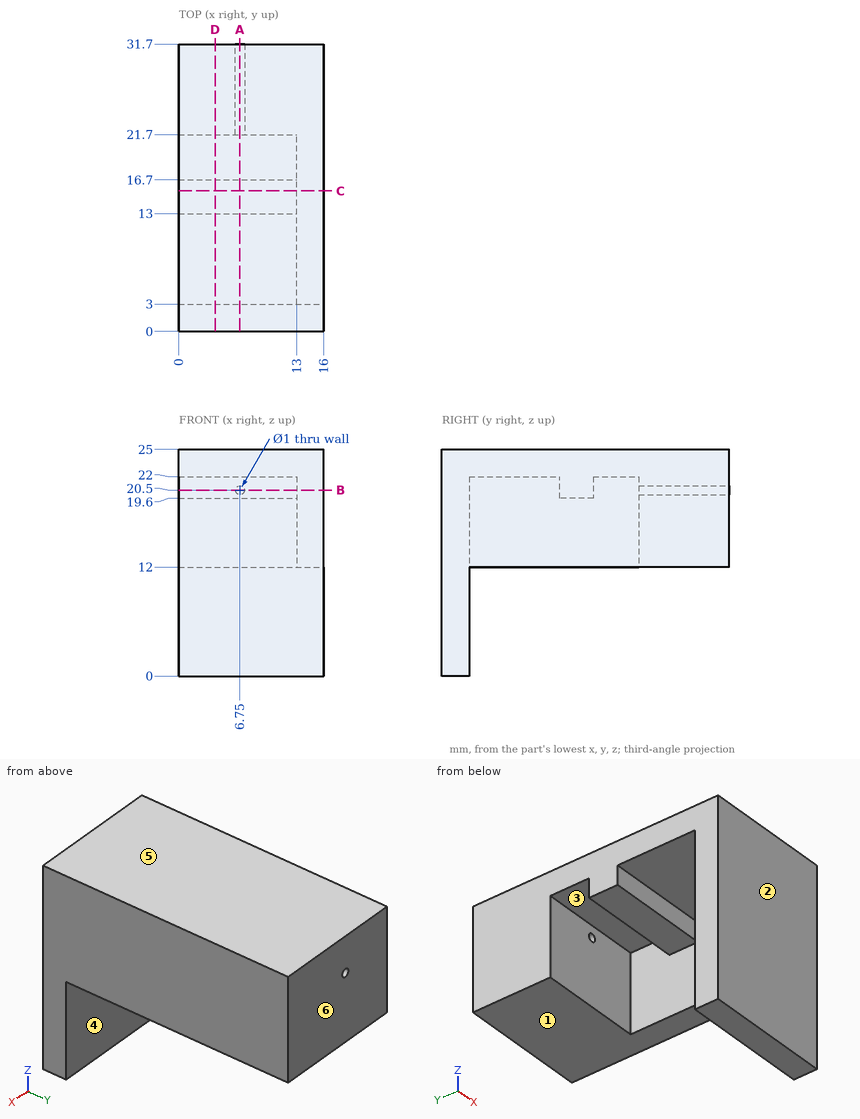
Can you work these out from the drawing? Everything is in mm from the part's minimum corner. A direction names the side the tool comes from. Give positions to 0.01 mm unless a question says otherwise; leave off trailing zeros. Order: outer loops, then holes, each group sorted by start corner. A loop starts at its lowest first (then second) coordinate and runs counter-clockwise, first axis right, second up. Notation, with made-up numbers: (-21.5, 17.5) -> (22.5, 17.5) arc R14 cw to (22.5, 40.5) -> close; hole circle Ø9 at (45, 70). An arc over 180 degrees is marked (long way). Return JSON: item names as keys, results as strings.
1. Imagine slicing it at C-C on y = 15.5. List the corners of the cut face in (x, z) for me.
Answer list:
{"outline": "(0, 19.6) -> (13, 19.6) -> (13, 12) -> (16, 12) -> (16, 25) -> (0, 25) -> close"}
2. For pin 1 Ø4 at (x, y) = (9, 15) entering from -Z; pin 2 Ø8 at (x, y) = (12.5, 18) entering from -Z; pin 3 Ø1 at (x, y) = (5.5, 11) entering from -Z, each with a flat end and sliding along its axis, tell me the tip position at first contact or that it passes through.
Answer list:
{"pin 1": "stops at z = 19.6", "pin 2": "stops at z = 12", "pin 3": "stops at z = 22"}
3. Thinking about a two-plate mould opening in Y: for the marked faces 4, 5 and 6, which applies, pulls with the +Y half, pulls with the -Y half, needs draft (parallel to the pull), parting line crosses it, or undercut?
Answer list:
{"face 4": "undercut", "face 5": "needs draft", "face 6": "pulls with the +Y half"}
4. I need wall thicknesses on line 1 (Y direction, x = 9.5, z = 20); line 2 (X direction, y = 25, z = 20.5); line 3 (Z direction, x = 6.75, y = 24). Which ranges of each line are inside material? Lowest first, please. Write a range as from..to.
Answer list:
{"line 1": "y = 0..3, 13..16.7, 21.7..31.7", "line 2": "x = 0..6.25, 7.25..16", "line 3": "z = 12..20, 21..25"}
5. Imagine slicing it at D-D on x = 4. List the corners of the cut face in (y, z) for me.
Answer list:
{"outline": "(0, 0) -> (3, 0) -> (3, 22) -> (13, 22) -> (13, 19.6) -> (16.7, 19.6) -> (16.7, 22) -> (21.7, 22) -> (21.7, 12) -> (31.7, 12) -> (31.7, 25) -> (0, 25) -> close"}
6. Imagine slicing it at B-B on z = 20.5. List the corners of the cut face in (x, y) for me, then the cut area to 3 significant figures.
Answer list:
{"outline": "(0, 0) -> (16, 0) -> (16, 31.7) -> (7.25, 31.7) -> (7.25, 21.7) -> (13, 21.7) -> (13, 16.7) -> (0, 16.7) -> (0, 13) -> (13, 13) -> (13, 3) -> (0, 3) -> close; (0, 21.7) -> (6.25, 21.7) -> (6.25, 31.7) -> (0, 31.7) -> close", "area": "302 mm2"}
7. On a 3-axis mill with a long thin cutter (end or side, diameter ignored), from which of +Z, -Z, +X, -X, +Y, -Y can I reach the whole of each face in a straight line? I mean the marked faces 1, 2 and 3. Say none if no direction works.
Answer list:
{"face 1": "-Z, +X, -X, +Y", "face 2": "+Z, -Z, +X, -X, -Y", "face 3": "-Z, -X"}
8. Imagine slicing it at A-A on x = 6.75. List the corners of the cut face in (y, z) for me.
Answer list:
{"outline": "(0, 0) -> (3, 0) -> (3, 22) -> (13, 22) -> (13, 19.6) -> (16.7, 19.6) -> (16.7, 22) -> (21.7, 22) -> (21.7, 21) -> (31.7, 21) -> (31.7, 25) -> (0, 25) -> close; (21.7, 12) -> (31.7, 12) -> (31.7, 20) -> (21.7, 20) -> close"}
